Geometry check sheet. Reference: the model listing, model coordinates, mm. A direction names the side the tool comes from. Coordinates: 2 decimals unless noted, no trailing zeros. Write each loop counter-clockwise with the first axis right and the second up, starting at its lowest first coordinate (ties: lowest second). Pieces come first, ordered by that corner, then holes.
from build123d import *

# Parameters (mm, degrees)
SKETCH_1_W         = 12.5
SKETCH_1_H         = 19.5
EXTRUDE_1_DEPTH    = 9
SKETCH_2_R         = 2.45
EXTRUDE_2_DEPTH    = 3
EXTRUDE_START      = 3
SKETCH_4_R         = 2.45
EXTRUDE_3_DEPTH    = 3
FILLET_1_R         = 0.25
HOLE_WIZARD_M6_1_D = 5
CHAMFER_1_SIZE     = 1


with BuildPart() as part:
    # 스케치1 → 보스-돌출1 (new body)
    with BuildSketch(Plane.XY):
        Rectangle(SKETCH_1_W, SKETCH_1_H)
    extrude(amount=EXTRUDE_1_DEPTH)

    # 스케치2 → 보스-돌출2 (add)
    with BuildSketch(Plane.XY.offset(9)):
        with Locations((0, 5.25)):
            Circle(SKETCH_2_R)
        with Locations((0, -4.75)):
            Circle(SKETCH_2_R)
    extrude(amount=EXTRUDE_2_DEPTH)

    # 스케치4 → 보스-돌출3 (add)
    with BuildSketch(Plane(origin=(0, 0, 0), x_dir=(-1, 0, 0), z_dir=(0, 0, -1)).offset(EXTRUDE_START)):
        with Locations(Location((0, -4.75, 0), (0, 0, 180))):
            Circle(SKETCH_4_R)
        with Locations(Location((0, 5.25, 0), (0, 0, 180))):
            Circle(SKETCH_4_R)
    extrude(amount=-EXTRUDE_3_DEPTH)

    # 필렛1
    fillet_1_edges = [part.edges().sort_by_distance(p)[0] for p in [
        (-2.45, -4.75, 12),
        (-2.45, 5.25, 12),
        (-2.45, -4.75, -3),
        (-2.45, 5.25, -3),
    ]]
    fillet(fillet_1_edges, radius=FILLET_1_R)

    # M6 탭을 위한 탭 드릴1 (through all)
    with Locations(Plane(origin=(0, -9.75, 4.5), x_dir=(0, 0, -1), z_dir=(0, -1, 0))):
        with Locations((0, 0)):
            Hole(HOLE_WIZARD_M6_1_D / 2)

    # 모따기1
    chamfer_1_edges = [part.edges().sort_by_distance(p)[0] for p in [
        (6.25, -9.75, 4.5),
        (-6.25, -9.75, 4.5),
        (-6.25, 9.75, 4.5),
        (6.25, 9.75, 4.5),
    ]]
    chamfer(chamfer_1_edges, length=CHAMFER_1_SIZE)


solid = part.part
1. Sectioned sample at C-C, the plane z = 6. Record the boundary of the cut face in (x, y), and give its area (3 significant figures).
Computed values:
outline: (-6.25, -8.75) - (-5.25, -9.75) - (-2, -9.75) - (-2, 9.75) - (-5.25, 9.75) - (-6.25, 8.75) - close; (2, -9.75) - (5.25, -9.75) - (6.25, -8.75) - (6.25, 8.75) - (5.25, 9.75) - (2, 9.75) - close
area: 164 mm2
2. Thickness scan on line 1 along X through (y, z) = (4, 4.5); line 2 along Z through (x, y) = (3.25, 6.5); line 3 along Y through (x, z) = (0, -2). Record the ranges inside material, lowest first.
Computed values:
line 1: x = -6.25 to -2.5, 2.5 to 6.25
line 2: z = 0 to 9
line 3: y = -7.2 to -2.3, 2.8 to 7.7
3. Access from +Z, -Z, +X, -X, +Y, -Y to the whole of each face (thin tool, end or side, straight path). Record for faces 4 (the cylindrical face through (-0.32, 2.82, -1.39)), 5 (the cylindrical face through (-0.32, -2.32, 10.36)), 6 (the flat face through (0, -5, 12)).
Computed values:
face 4: -Z
face 5: +Z
face 6: +Z, +X, -X, +Y, -Y
4. Sectioned sample at D-D, the plane z = 4.5. Record the boundary of the cut face in (x, y).
Computed values:
outline: (-6.25, -8.75) - (-5.25, -9.75) - (-2.5, -9.75) - (-2.5, 9.75) - (-5.25, 9.75) - (-6.25, 8.75) - close; (2.5, -9.75) - (5.25, -9.75) - (6.25, -8.75) - (6.25, 8.75) - (5.25, 9.75) - (2.5, 9.75) - close
5. Draft check along Y on faces 1 (the cylindrical face through (-0.53, 2.86, 10.36)), 2 (the flat face through (0, 5, -3)), 3 (the flat face through (-6, 9, 4)). Enter one of: released by +Y, released by -Y, zero draft, split by the parting line, or undercut.
Computed values:
face 1: undercut
face 2: zero draft
face 3: released by +Y
6. Sectioned sample at A-A, the plane y = -4.75. Record the boundary of the cut face in (x, z).
Computed values:
outline: (-6.25, 0) - (-2.45, 0) - (-2.45, -2.75) arc R0.25 ccw to (-2.2, -3) - (2.2, -3) arc R0.25 ccw to (2.45, -2.75) - (2.45, 0) - (6.25, 0) - (6.25, 9) - (2.45, 9) - (2.45, 11.75) arc R0.25 ccw to (2.2, 12) - (-2.2, 12) arc R0.25 ccw to (-2.45, 11.75) - (-2.45, 9) - (-6.25, 9) - close; hole circle Ø5 at (0, 4.5)
